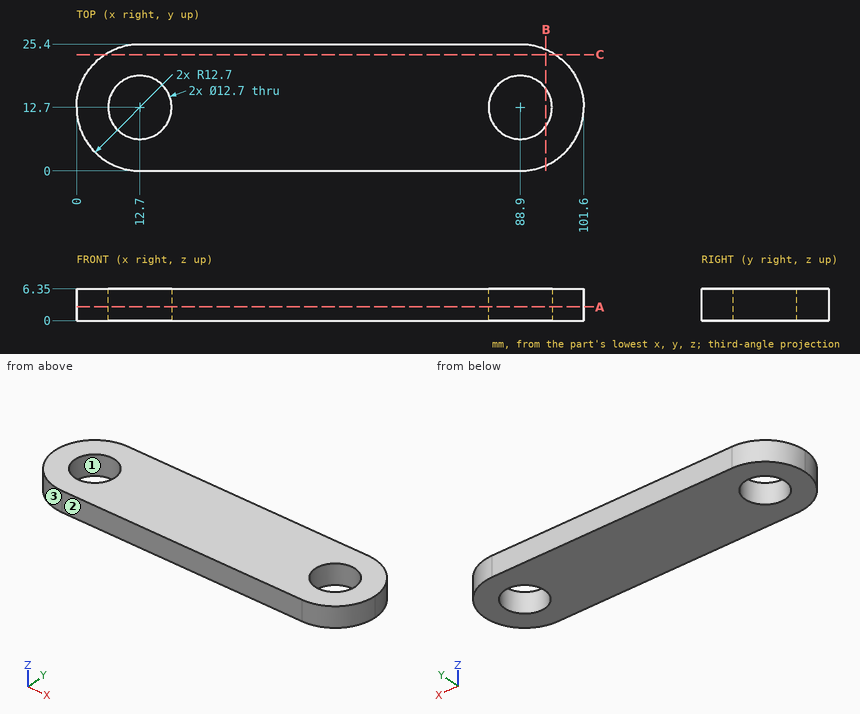
Answer from the drawing. Dimensions are ordinates in mm from the lowest x, y and z of the part. Round coordinates to 2 decimals unless told otherwise and drop trailing zeros. Loops run counter-clockwise (first coordinate to the right, second up) from the corner with the lowest first, then second, coordinate; pieces in that order, holes last. Notation, with made-up numbers: (19, 86.5) - (51, 86.5) arc R17 ccw to (51, 107.5) - close; hole circle Ø2 at (-11.75, 73). An arc over 180 degrees is marked (long way). Return JSON: item names as keys, results as strings. Group by question number.
1. Each of these flat-tipped pins is pushed along its axis until it touches: P1, Ø3, axis at y = 5, z = 3.5, coming from the +X side; P2, Ø1.5, axis at y = 14, z = 1.5, coming from the +X side; P3, Ø1.5, axis at y = 8.5, z = 5.5, coming from the -X side. Where does it stop, or does it pass through?
2. The part is cut by section B-B on x = 94. Determine the outline of the cut face in (y, z), then the cut area to 3 significant figures.
3. Consider probe 1 along X at (y, z) = (14.5, 1); probe 2 along X at (y, z) = (18, 0.75); probe 3 along Y at (x, z) = (88.9, 2.25). Determine where each line is inside the solid, lowest interval first.
4. The mould has two halves that part along X. Classify the marked faces 1, 2 and 3: pulls with the +X half, pulls with the -X half, needs draft (parallel to the pull), parting line crosses it, or undercut.
5. The part is cut by section A-A on z = 2.75. State how many separate pieces and enclosed holes the cut face has, then the cut area to 3 significant figures.
6. The part is cut by section C-C on y = 23.25. Determine the outline of the cut face in (x, z).
Resolved:
{
 "1": {"P1": "stops at x = 99.98", "P2": "stops at x = 101.59", "P3": "stops at x = 0.48"},
 "2": {"outline": "(1.07, 0) - (8.92, 0) - (8.92, 6.35) - (1.07, 6.35) - close; (16.48, 0) - (24.33, 0) - (24.33, 6.35) - (16.48, 6.35) - close", "area": "99.7 mm²"},
 "3": {"probe 1": "x = 0.13 to 6.61, 18.79 to 82.81, 94.99 to 101.47", "probe 2": "x = 1.16 to 9.2, 16.2 to 85.4, 92.4 to 100.44", "probe 3": "y = 0 to 6.35, 19.05 to 25.4"},
 "4": {"face 1": "undercut", "face 2": "needs draft", "face 3": "pulls with the -X half"},
 "5": {"separate pieces": "1", "enclosed holes": "2", "area": "2,190 mm²"},
 "6": {"outline": "(5.63, 0) - (95.97, 0) - (95.97, 6.35) - (5.63, 6.35) - close"}
}
